Geometry: final body of the model. Coordinates: model frame, mm. Face numbers are marked on the shaded views. A direction names the side the tool comes from. Give positions to 0.01 mm unless a question says otherwise; leave off trailing zeros. Loops run counter-clockwise (first coordinate to the right, second up) from the corner with the lowest first, then second, coordinate; pieces in that order, holes last. Notation, with made-up numbers: M -21,-19 L -8,-19 A22 cw -8,-13 Z; hole C 31.25,54.25 d5. An arc over 180 degrees is marked long. Put each result on its own line as item: value.
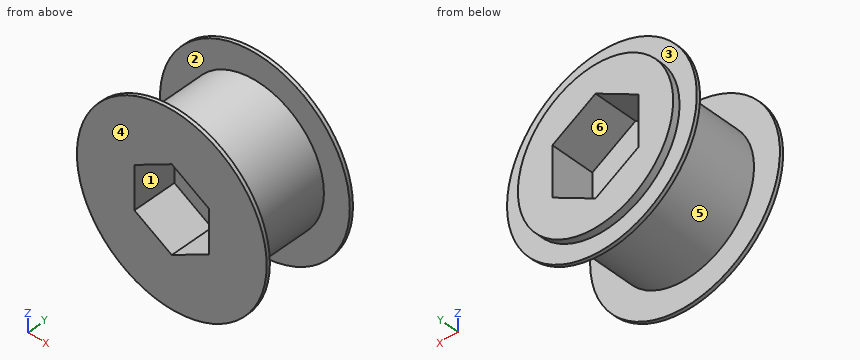
```python
from build123d import *

# Parameters (mm, degrees)
F0_R      = 5.08
F1_DEPTH  = 6.35
F2_R      = 6.985
F3_DEPTH  = 0.254
F4_R      = 6.985
F5_DEPTH  = 0.254
F7_DEPTH  = 3.175
F8_R      = 5.715
F9_DEPTH  = 0.508
F11_DEPTH = 3.175


with BuildPart() as f1:
    # F0 (on Front) → F1 (new body)
    with BuildSketch(Plane.XZ):
        Circle(F0_R)
    extrude(amount=F1_DEPTH)

    # F2 (on face) → F3 (join)
    with BuildSketch(Plane.XZ.offset(6.35)):
        Circle(F2_R)
    extrude(amount=F3_DEPTH)

    # F4 (on Front) → F5 (join)
    with BuildSketch(Plane.XZ):
        Circle(F4_R)
    extrude(amount=-F5_DEPTH)

    # F6 (on face) → F7 (cut)
    with BuildSketch(Plane.XZ.offset(6.604)):
        Polygon((0, 3.175), (-2.749630657, 1.5875), (-2.749630657, -1.5875), (0, -3.175), (2.749630657, -1.5875), (2.749630657, 1.5875), align=None)
    extrude(amount=-F7_DEPTH, mode=Mode.SUBTRACT)

    # F8 (on face) → F9 (join)
    with BuildSketch(Plane(origin=(0, 0.254, 0), x_dir=(-1, 0, 0), z_dir=(0, 1, 0))):
        Circle(F8_R)
    extrude(amount=F9_DEPTH)

    # F10 (on face) → F11 (cut)
    with BuildSketch(Plane(origin=(0, 0.762, 0), x_dir=(-1, 0, 0), z_dir=(0, 1, 0))):
        Polygon((-3.175, 1.8330871047), (-3.175, -1.8330871047), (0, -3.6661742094), (3.175, -1.8330871047), (3.175, 1.8330871047), (0, 3.6661742094), align=None)
    extrude(amount=-F11_DEPTH, mode=Mode.SUBTRACT)


solid = f1.part
```
Item 1: Mould query, pull axis Z, two halves, no side actions, for the marked faces 4, 5 and 6. Classes: pulls with the +Z half, pulls with the -Z half, needs draft (parallel to the pull), parting line crosses it, or undercut.
Output values:
face 4: needs draft
face 5: parting line crosses it
face 6: undercut
Item 2: Section B-B on z = -5.25. Output: boundary loops of the cut face in (x, y), then the cut area to 3 significant figures.
Output values:
outline: M -4.61,-6.6 L 4.61,-6.6 L 4.61,-6.35 L -4.61,-6.35 Z; M -4.61,0 L 4.61,0 L 4.61,0.25 L 2.26,0.25 L 2.26,0.76 L -2.26,0.76 L -2.26,0.25 L -4.61,0.25 Z
area: 6.98 mm²
Item 3: Section A-A on y = -5. Output: boundary loops of the cut face in (x, z) (1 decimal), then the cut area to 3 significant figures.
Output values:
outline: C 0,0 d10.2; hole M -2.7,-1.6 L 0,-3.2 L 2.7,-1.6 L 2.7,1.6 L 0,3.2 L -2.7,1.6 Z
area: 54.9 mm²
Item 4: Line query: probe 1 along Y at (x, z) = (-4.25, 4); probe 2 along Y at (x, z) = (0.5, 5.25); probe 3 along Y at (x, z) = (0.5, 2). Output: solid intervals per line, ascending. Write a range as [from, to].
Output values:
probe 1: [-6.6, -6.35], [0, 0.25]
probe 2: [-6.6, -6.35], [0, 0.76]
probe 3: [-3.43, -2.41]
Item 5: Section C-C on x = -5.5. Output: boundary loops of the cut face in (y, z), then the cut area to 3 significant figures.
Output values:
outline: M -6.6,-4.31 L -6.35,-4.31 L -6.35,4.31 L -6.6,4.31 Z; M 0,-4.31 L 0.25,-4.31 L 0.25,-1.55 L 0.76,-1.55 L 0.76,1.55 L 0.25,1.55 L 0.25,4.31 L 0,4.31 Z
area: 5.95 mm²
Item 6: Section D-D on z = 0. Output: boundary loops of the cut face in (x, y) (3 decimals).
Output values:
outline: M -6.985,-6.604 L -2.75,-6.604 L -2.75,-3.429 L 2.75,-3.429 L 2.75,-6.604 L 6.985,-6.604 L 6.985,-6.35 L 5.08,-6.35 L 5.08,0 L 6.985,0 L 6.985,0.254 L 5.715,0.254 L 5.715,0.762 L 3.175,0.762 L 3.175,-2.413 L -3.175,-2.413 L -3.175,0.762 L -5.715,0.762 L -5.715,0.254 L -6.985,0.254 L -6.985,0 L -5.08,0 L -5.08,-6.35 L -6.985,-6.35 Z
Item 7: Pin query (flat end, axial travel): pin 1 Ø4.5 at (x, z) = (0, 0.5) entering from -Y; pin 2 Ø3.5 at (y, z) = (-4.5, 0.5) entering from -X; pin 3 Ø1 at (y, z) = (-5, 0.5) entering from +X. Return the tip coordinate at first contact, or that it passes through.
Output values:
pin 1: y = -3.43
pin 2: x = -5.08
pin 3: x = 5.08
Item 8: Set-up query: the marked faces 1, 2 and 3. Return all of +Z, -Z, +X, -X, +Y, -Y with unobstructed straight access to the full face (end or side cutting, diameter ignored); none if empty.
Output values:
face 1: -Y
face 2: none
face 3: +Y
